The listing builds one solid part. Answer for the finished solid, in the listing's coordinates (mm). Face numbers are marked on the shaded views. Coordinates: 2 decimals unless noted, no trailing zeros. Loops run counter-clockwise (first coordinate to the right, second up) from the corner with the lowest first, then second, coordinate; pieces in that order, holes last. Notation, with made-up numbers: M 18,-12 L 69,-12 A29 ccw 69,19 Z; hole C -32.5,81.25 d10. An arc over 180 degrees is marked long. Answer in a Markdown table with one row per item. Add a question column.
from build123d import *

# Parameters (mm, degrees)
SKETCH_R      = 18
SKETCH_R_2    = 13.5
PAD_DEPTH     = 3
SKETCH001_R   = 15.4
SKETCH001_R_2 = 1.55
PAD001_DEPTH  = 3
FILLET_R      = 1


with BuildPart() as part:
    # Sketch → Pad (new body)
    with BuildSketch(Plane.XY):
        Circle(SKETCH_R)
        Circle(SKETCH_R_2, mode=Mode.SUBTRACT)
    extrude(amount=PAD_DEPTH)

    # Sketch001 (on Face4 of Pad) → Pad001 (join)
    with BuildSketch(Plane.XY.offset(3)):
        with BuildLine():
            ThreePointArc((-16.124515, -8), (0, -18), (16.124515, -8))
            Line((24.325621, -2.986153), (16.124515, -8))
            ThreePointArc((24.325621, -2.986153), (26, 0), (24.325621, 2.986153))
            Line((24.325621, 2.986153), (16.124515, 8))
            ThreePointArc((16.124515, 8), (0, 18), (-16.124515, 8))
            Line((-24.325621, 2.986153), (-16.124515, 8))
            ThreePointArc((-24.325621, 2.986153), (-26, 0), (-24.325621, -2.986153))
            Line((-24.325621, -2.986153), (-16.124515, -8))
        make_face()
        Circle(SKETCH001_R, mode=Mode.SUBTRACT)
        with Locations((-22.5, 0)):
            Circle(SKETCH001_R_2, mode=Mode.SUBTRACT)
        with Locations((22.5, 0)):
            Circle(SKETCH001_R_2, mode=Mode.SUBTRACT)
    extrude(amount=PAD001_DEPTH)

    # Fillet
    fillet_edges = [part.edges().sort_by_distance(p)[0] for p in [
        (-15.4, 0, 3),
    ]]
    fillet(fillet_edges, radius=FILLET_R)


solid = part.part
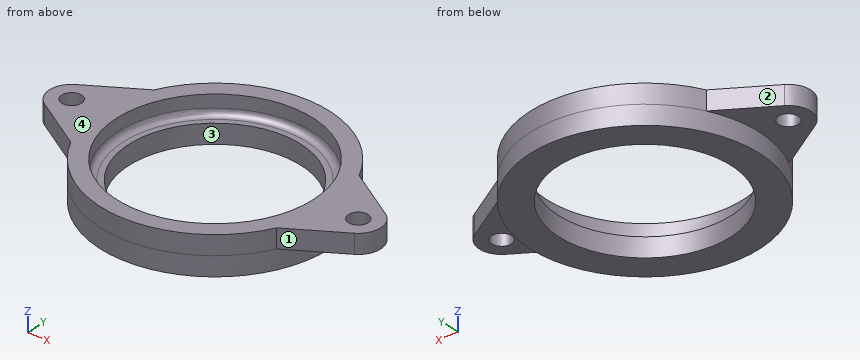
(1) A cutting plane is placed at B-B (y = 0). Give the vertices of the cut face in (x, z), plus the area to 3 significant figures.
(2) Straight lines are drawn through the part: line 1 (Y direction, x = 0, z = 2.1); line 2 (Y direction, x = -22.5, z = 4.4); line 3 (X direction, y = 11.5, z = 3.9). For each, find the intervals that lie inside material, in ascending order.
(3) Each of these flat-tipped pins is pushed along its axis until it touches: pin 1 (1.5 mm diameter, centred on x = 10, z = 5, fed in from -Y); pin 2 (4 mm diameter, centred on x = 22.5, y = 0, fed in from -Z); pin 3 (1 mm diameter, centred on y = -2, z = 1.5, fed in from -X); pin 4 (8 mm diameter, centred on x = 19, y = -12, fed in from +Z). Where does it stop, or does it pass through?
(4) A cutting plane is placed at C-C (z = 1.15). Give the vertices of the cut face in (x, y), plus the area to 3 significant figures.
(5) The mould has two halves that part along Y. Classify the marked faces 1, 2, 3 and 4: released by +Y, released by -Y, zero draft, split by the parting line, or undercut.
(6) A cutting plane is placed at D-D (x = 22.5). Give the vertices of the cut face in (y, z), plus the area to 3 significant figures.
(7) A cutting plane is placed at A-A (x = 0). Give the vertices of the cut face in (y, z), plus the area to 3 significant figures.
Solved:
| question | item | result |
|---|---|---|
| 1 | outline | M -26,3 L -24.05,3 L -24.05,6 L -26,6 Z; M -20.95,3 L -18,3 L -18,0 L -13.5,0 L -13.5,3 L -14.4,3 A1 cw -15.4,4 L -15.4,6 L -20.95,6 Z; M 13.5,0 L 18,0 L 18,3 L 20.95,3 L 20.95,6 L 15.4,6 L 15.4,4 A1 cw 14.4,3 L 13.5,3 Z; M 24.05,3 L 26,3 L 26,6 L 24.05,6 Z |
| 1 | area | 72.4 mm² |
| 2 | line 1 | y = -18 to -13.5, 13.5 to 18 |
| 2 | line 2 | y = -4.1 to -1.55, 1.55 to 4.1 |
| 2 | line 3 | x = -13.85 to -10.24, 10.24 to 13.85 |
| 3 | pin 1 | stops at y = -15.44 |
| 3 | pin 2 | stops at z = 3 |
| 3 | pin 3 | stops at x = -17.94 |
| 3 | pin 4 | passes through |
| 4 | outline | C 0,0 d36; hole C 0,0 d27 |
| 4 | area | 445 mm² |
| 5 | face 1 | released by -Y |
| 5 | face 2 | released by +Y |
| 5 | face 3 | undercut |
| 5 | face 4 | zero draft |
| 6 | outline | M -4.1,3 L -1.55,3 L -1.55,6 L -4.1,6 Z; M 1.55,3 L 4.1,3 L 4.1,6 L 1.55,6 Z |
| 6 | area | 15.3 mm² |
| 7 | outline | M -18,0 L -13.5,0 L -13.5,3 L -14.4,3 A1 cw -15.4,4 L -15.4,6 L -18,6 Z; M 13.5,0 L 18,0 L 18,6 L 15.4,6 L 15.4,4 A1 cw 14.4,3 L 13.5,3 Z |
| 7 | area | 43.0 mm² |
